Geometry: final body of the model. Coordinates: model frame, mm. Face numbers are marked on the shaded views. Round coordinates to 2 decimals unless told otherwise and drop trailing zeros. Order: outer loops, then holes, each group sorted by start corner. A loop starts at its lowest first (then second) coordinate and runs counter-clockwise, first axis right, second up. Notation, with made-up numbers: M 56,21.25 L 85,21.25 A23 ccw 85,36.25 Z; hole C -24,5.5 d10. An arc over 180 degrees is marked long. Put each result on its own line as item: value. Start each with the question number.
1) Section A-A, the plane z = 0. Return loops of the section in (x, y).
2) Section B-B, the plane x = 0. Return loops of the section in (y, z), then the cut area to 3 significant figures.
3) First-contact query: P1, Ø3.5, axis at x = 2, y = 1, coming from the +Z side; P2, Ø1.5, axis at y = 1.5, z = 14.5, coming from the +X side; P3, Ø5, axis at y = 11, z = -36, coming from the -X side. Flat tips, straight axial feed; report the tip coordinate or a pass-through.
4) Section C-C, the plane y = 11.75. Return loops of the section in (x, z), then the cut area to 3 significant figures.
5) Draft query along Z for the marked faces 1, 2, 3 and 4. Return one class per face: pulls with the +Z half, pulls with the -Z half, needs draft (parallel to the pull), parting line crosses it, or undercut.
6) Section D-D, the plane x = -34. Return loops of the section in (y, z), then the cut area to 3 significant figures.
7) Material intervals for probe 1 along X at (y, z) = (7, 0); probe 2 along Z at (x, y) = (1, 4.5); probe 3 along Y at (x, z) = (-24.5, -21), sorted ascending. Write a range as [from, to].
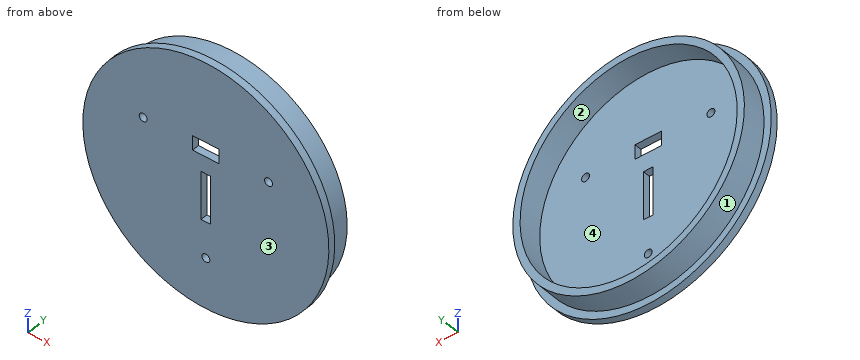
from build123d import *

# Parameters (mm, degrees)
SKETCH_1_R               = 51
EXTRUDE_1_DEPTH          = 3
SKETCH_2_R               = 48
SKETCH_2_R_2             = 45
EXTRUDE_2_DEPTH          = 10
SKETCH_5_R               = 1.65
CUT_EXTRUDE_1_DEPTH      = 10
PATTERN_CIRCULAR_1_COUNT = 3
SKETCH_6_W               = 4
SKETCH_6_H               = 20
SKETCH_6_W_2             = 11
SKETCH_6_H_2             = 6
CUT_EXTRUDE_2_DEPTH      = 10


with BuildPart() as part:
    # Эскиз1 → Бобышка-Вытянуть1 (new body)
    with BuildSketch(Plane(origin=(0, 0, 0), x_dir=(1, 0, 0), z_dir=(0, 1, 0))):
        with Locations(Location((0, 0, 0), (0, 0, 270))):
            Circle(SKETCH_1_R)
    extrude(amount=EXTRUDE_1_DEPTH)

    # Эскиз2 → Бобышка-Вытянуть2 (add)
    with BuildSketch(Plane(origin=(0, 3, 0), x_dir=(1, 0, 0), z_dir=(0, 1, 0))):
        with Locations(Location((0, 0, 0), (0, 0, 270))):
            Circle(SKETCH_2_R)
        with Locations(Location((0, 0, 0), (0, 0, 270))):
            Circle(SKETCH_2_R_2, mode=Mode.SUBTRACT)
    extrude(amount=EXTRUDE_2_DEPTH)

    # Эскиз5 → Вырез-Вытянуть1 (cut)
    with BuildSketch(Plane(origin=(0, 3, 0), x_dir=(1, 0, 0), z_dir=(0, 1, 0))):
        with Locations(Location((0, 30, 0), (0, 0, 270))):
            Circle(SKETCH_5_R)
    cut_extrude_1 = extrude(amount=-CUT_EXTRUDE_1_DEPTH, mode=Mode.SUBTRACT)

    # Круговой массив1: Вырез-Вытянуть1 ×3 about axis
    pattern_circular_1_axis = Axis((0, 0, 0), (0, 1, 0))
    for i in range(1, PATTERN_CIRCULAR_1_COUNT):
        add(cut_extrude_1.rotate(pattern_circular_1_axis, i * 360 / PATTERN_CIRCULAR_1_COUNT), mode=Mode.SUBTRACT)

    # Эскиз6 → Вырез-Вытянуть2 (cut)
    with BuildSketch(Plane(origin=(0, 3, 0), x_dir=(1, 0, 0), z_dir=(0, 1, 0))):
        with Locations((0, 5)):
            Rectangle(SKETCH_6_W, SKETCH_6_H)
        with Locations((0, -15)):
            Rectangle(SKETCH_6_W_2, SKETCH_6_H_2)
    extrude(amount=-CUT_EXTRUDE_2_DEPTH, mode=Mode.SUBTRACT)


solid = part.part
Result sheet:
1. outline: M -51,0 L -2,0 L -2,3 L -45,3 L -45,13 L -48,13 L -48,3 L -51,3 Z; M 2,0 L 51,0 L 51,3 L 48,3 L 48,13 L 45,13 L 45,3 L 2,3 Z
2. outline: M 0,-51 L 3,-51 L 3,-48 L 13,-48 L 13,-45 L 3,-45 L 3,-31.65 L 0,-31.65 Z; M 0,-28.35 L 3,-28.35 L 3,-15 L 0,-15 Z; M 0,5 L 3,5 L 3,12 L 0,12 Z; M 0,18 L 3,18 L 3,45 L 13,45 L 13,48 L 3,48 L 3,51 L 0,51 Z
2. area: 278 mm2
3. P1: stops at z = 51
3. P2: stops at x = 49.11
3. P3: stops at x = -34.38
4. outline: C 0,0 d96; hole C 0,0 d90
4. area: 877 mm2
5. face 1: parting line crosses it
5. face 2: undercut
5. face 3: needs draft
5. face 4: undercut
6. outline: M 0,-38.01 L 3,-38.01 L 3,-33.88 L 13,-33.88 L 13,-29.48 L 3,-29.48 L 3,29.48 L 13,29.48 L 13,33.88 L 3,33.88 L 3,38.01 L 0,38.01 Z
6. area: 316 mm2
7. probe 1: x = [-48, -45], [45, 48]
7. probe 2: z = [-47.99, -44.99], [44.99, 47.99]
7. probe 3: y = [0, 3]
